from build123d import *

# Parameters (mm, degrees)
F1_DEPTH = 6


with BuildPart() as f1:
    # F0 (on Front) → F1 (new body)
    with BuildSketch(Plane.XZ):
        Polygon((144, 57.272727), (144, 70), (-144, 70), (-144, 57.272727), (-150, 57.272727), (-150, 44.545455), (-144, 44.545455), (-144, 37.818182), (-144, 31.818182), (-150, 31.818182), (-150, 19.090909), (-144, 19.090909), (-144, 12.363636), (-144, 6.363636), (-150, 6.363636), (-150, -6.363636), (-144, -6.363636), (-144, -13.090909), (-144, -19.090909), (-150, -19.090909), (-150, -31.818182), (-144, -31.818182), (-144, -38.545455), (-144, -44.545455), (-150, -44.545455), (-150, -57.272727), (-144, -57.272727), (-144, -64), (-135.714286, -64), (-135.714286, -70), (-121.428571, -70), (-121.428571, -64), (-107.142857, -64), (-107.142857, -70), (-92.857143, -70), (-92.857143, -64), (-78.571429, -64), (-78.571429, -70), (-64.285714, -70), (-64.285714, -64), (-50, -64), (-50, -70), (-35.714286, -70), (-35.714286, -64), (-21.428571, -64), (-21.428571, -70), (-7.142857, -70), (-7.142857, -64), (7.142857, -64), (7.142857, -70), (21.428571, -70), (21.428571, -64), (35.714286, -64), (35.714286, -70), (50, -70), (50, -64), (64.285714, -64), (64.285714, -70), (78.571429, -70), (78.571429, -64), (92.857143, -64), (92.857143, -70), (107.142857, -70), (107.142857, -64), (121.428571, -64), (121.428571, -70), (135.714286, -70), (135.714286, -64), (144, -64), (144, -57.272727), (150, -57.272727), (150, -44.545455), (144, -44.545455), (144, -38.545455), (144, -31.818182), (150, -31.818182), (150, -19.090909), (144, -19.090909), (144, -13.090909), (144, -6.363636), (150, -6.363636), (150, 6.363636), (144, 6.363636), (144, 12.363636), (144, 19.090909), (150, 19.090909), (150, 31.818182), (144, 31.818182), (144, 37.818182), (144, 44.545455), (150, 44.545455), (150, 57.272727), align=None)
    extrude(amount=F1_DEPTH)


solid = f1.part
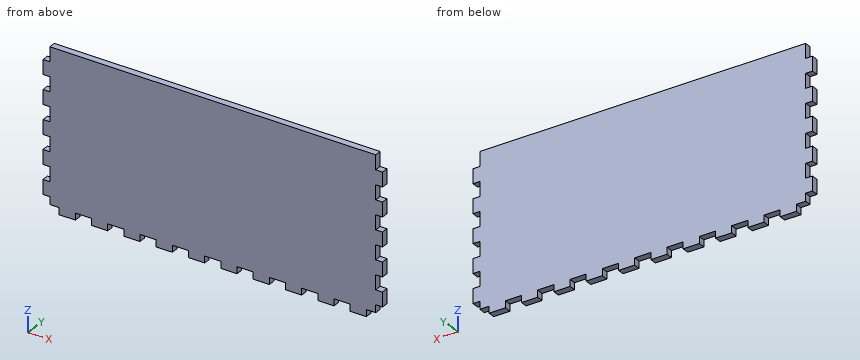
Can you work these out from the model? Positions are in its coordinate system, mm. Round coordinates to 2 decimals unless told otherwise and drop trailing zeros. Order: outer loops, then holes, each group sorted by start corner. A loop starts at its lowest first (then second) coordinate and runs counter-clockwise, first axis right, second up. Notation, with made-up numbers: (-18.75, 17) -> (2.25, 17) arc R11 ccw to (2.25, 37) -> close; hole circle Ø7 at (-9.5, 45.5). An arc over 180 degrees is marked (long way). Write each question's results on one line, items separated by ' | '. Start each with the question number.
Item 1: Will these pins go through, and if not, where does the flat tip stop? pin 1 (1.8 mm diameter, centred on x = 146.5, y = -4, fed in from -Z); pin 2 (3 mm diameter, centred on x = -147, y = -3.5, fed in from +Z); pin 3 (1.8 mm diameter, centred on y = -3.5, z = -66, fed in from +X).
Item 2: Please list where these lines run through material, in increasing order: L1, parallel to X at y = -4.55, z = -42.5; L2, parallel to Z at x = 29, y = -2.95.
Item 3: If we section it at B-B, the plane z = -16: Write out the boundary of the cut face in (x, y).
Item 4: If we section it at A-A, the plane x = 56: Write out the boundary of the cut face in (y, z), then the cut area to 3 significant figures.
Results:
1) pin 1: stops at z = -57.27 | pin 2: stops at z = 57.27 | pin 3: stops at x = 135.71
2) L1: x = -144 to 144 | L2: z = -64 to 70
3) outline: (-144, -6) -> (144, -6) -> (144, 0) -> (-144, 0) -> close
4) outline: (-6, -64) -> (0, -64) -> (0, 70) -> (-6, 70) -> close | area: 804 mm2
